Design review of the part built by this model. Coordinates are the model's own, in mm. Face numbers are marked on the shaded views. A direction names the side the tool comes from. Round coordinates to 2 decimals unless told otherwise and drop trailing zeros. Loops run counter-clockwise (first coordinate to the right, second up) from the corner with the lowest first, then second, coordinate; pieces in that order, holes last. Notation, with made-up numbers: (-15, -10.75) - (26, -10.75) arc R34 cw to (26, 20.25) - close; hole circle Ø1 at (80.5, 21). An arc over 180 degrees is marked (long way). Answer as CSV lines item,"result". Start each with the question number.
(1) For the marked faces 4, 5 and 6, list the 3-axis set-ups (+Z, -Z, +X, -X, +Y, -Y) from which the entire face can be reached by the end or side of a thin tool; tool diameter is ignored.
(2) For P1, Ø1.5, axis at x = -2, z = 6, coming from the -Y side; P2, Ø0.6, axis at x = 13, z = 4.5, coming from the -Y side; P3, Ø1.1, axis at x = 1.5, z = 6.5, coming from the +Y side, all flat-tipped, find the tip position at first contact; note any pin that passes through.
(3) Wall thickness on L1, parallel to X at y = 0, z = 1.75; L2, parallel to Y at x = 0, z = 1.25; L3, parallel to Y at x = 0, z = 5.65: over which ranges is each line inside the solid? List them lowest first.
(4) Consider section D-D (x = 5). Give the boundary of the cut face in (y, z), and give its area (3 significant figures).
(5) Consider section B-B (x = 10). Give the boundary of the cut face in (y, z), and give its area (3 significant figures).
(6) Consider section A-A (z = 2). Give the boundary of the cut face in (x, y).
(7) Consider section C-C (x = 0). Give the boundary of the cut face in (y, z) (3 decimals), and give its area (3 significant figures).
(8) Mouldability with a two-part tool opening along Z and no side actions: class the marked faces 1, 2 and 3 as released by +Z, released by -Z, zero draft, split by the parting line, or undercut.
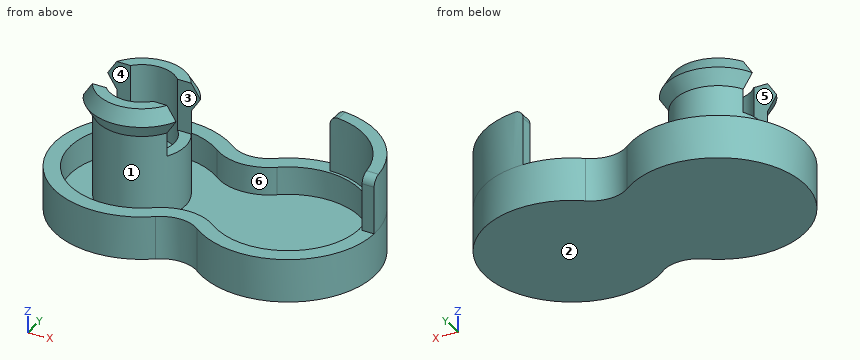
from build123d import *
from build123d.topology import SkipClean

# Parameters (mm, degrees)
BOSS_EXTRUDE1_DEPTH = 2.5
SHELL1_T            = -0.88
BOSS_EXTRUDE2_DEPTH = 3.25
FILLET1_R           = 0.5
FILLET2_R           = 0.5
SKETCH3_R           = 2.5
BOSS_EXTRUDE3_DEPTH = 6.5
SKETCH5_R           = 1.85
CUT_EXTRUDE1_DEPTH  = 4.22
SKETCH8_W           = 6.47168307
SKETCH8_H           = 2.5
CUT_EXTRUDE2_DEPTH  = 3
SKETCH9_W           = 5
SKETCH9_H           = 5
CUT_EXTRUDE3_DEPTH  = 3.25


# Read off the part's stored shape, not the designer's step: Mirror1
with BuildPart() as part:
    # Sketch1 → Boss-Extrude1 (new body)
    with BuildSketch(Plane.XY):
        with BuildLine():
            ThreePointArc((3.035714286, 3.972963475), (-5, 0), (3.035714286, -3.972963475))
            ThreePointArc((3.035714286, -3.972963475), (4.25, -3.562148865), (5.464285714, -3.972963475))
            ThreePointArc((5.464285714, -3.972963475), (13.5, 0), (5.464285714, 3.972963475))
            ThreePointArc((5.464285714, 3.972963475), (4.25, 3.562148865), (3.035714286, 3.972963475))
        make_face()
    extrude(amount=BOSS_EXTRUDE1_DEPTH)

    # Shell1
    shell1_openings = [part.faces().sort_by_distance(p)[0] for p in [
        (4.25, 0, 2.5),
    ]]
    offset(amount=SHELL1_T, openings=shell1_openings, kind=Kind.INTERSECTION)

    # Sketch2 → Boss-Extrude2 (add)
    with BuildSketch(Plane.XY.offset(2.5)):
        with BuildLine():
            Line((13.5, 0), (12.8, 0))
            ThreePointArc((12.8, 0), (11.540559159, -3.040559159), (8.5, -4.3))
            Line((8.5, -4.3), (8.5, -5))
            ThreePointArc((8.5, -5), (12.035533906, -3.535533906), (13.5, 0))
        make_face()
    extrude(amount=BOSS_EXTRUDE2_DEPTH)

    # Fillet1
    fillet1_edges = [part.edges().sort_by_distance(p)[0] for p in [
        (8.5, -4.65, 5.75),
    ]]
    fillet(fillet1_edges, radius=FILLET1_R)

    # Fillet2
    fillet2_edges = [part.edges().sort_by_distance(p)[0] for p in [
        (13.15, 0, 5.75),
    ]]
    fillet(fillet2_edges, radius=FILLET2_R)

    # Sketch3 → Boss-Extrude3 (add)
    with BuildSketch(Plane.XY.offset(0.88)):
        with Locations(Location((0, 0, 0), (0, 0, 180))):
            Circle(SKETCH3_R)
    extrude(amount=BOSS_EXTRUDE3_DEPTH)

    # Sketch5 → Cut-Extrude1 (cut)
    with BuildSketch(Plane.XY.offset(7.38)):
        Circle(SKETCH5_R)
    extrude(amount=-CUT_EXTRUDE1_DEPTH, mode=Mode.SUBTRACT)

    # Sketch6 → Revolve1 (revolve)
    with BuildSketch(Plane(origin=(0, 0, 0), x_dir=(1, 0, 0), z_dir=(0, 1, 0))):
        Polygon((2.5, -5.75), (2.5, -7.38), (2.970540469, -6.565), align=None)
    revolve(axis=Axis((0, 0, 7.38), (0, 0, -1)))

    # Sketch8 → Cut-Extrude2 (cut)
    with BuildSketch(Plane.XY.offset(7.38)):
        Rectangle(SKETCH8_W, SKETCH8_H)
    extrude(amount=-CUT_EXTRUDE2_DEPTH, mode=Mode.SUBTRACT)

    # Mirror1: part across plane


with BuildPart() as part_1:
    with SkipClean():  # the faces are left unmerged after this step: merging them gives an invalid solid
        add(part.part)
        add(part.part.mirror(Plane.ZX))

    # Sketch9 → Cut-Extrude3 (cut)
    with SkipClean():  # the faces are left unmerged after this step: merging them gives an invalid solid
        with BuildSketch(Plane.XY.offset(5.75)):
            with Locations((11, -2.5)):
                Rectangle(SKETCH9_W, SKETCH9_H)
        extrude(amount=-CUT_EXTRUDE3_DEPTH, mode=Mode.SUBTRACT)


solid = part_1.part
Determined:
1,face 4,"+Z, -X"
1,face 5,"+Z, +X, -X"
1,face 6,"+Z"
2,P1,"stops at y = -2.56"
2,P2,"stops at y = 0"
2,P3,"stops at y = 2.81"
3,L1,"x = -5 to -4.12, -2.5 to 2.5, 12.62 to 13.5"
3,L2,"y = -5 to -4.12, -2.5 to 2.5, 4.12 to 5"
3,L3,"y = -2.5 to -1.85, 1.85 to 2.5"
4,outline,"(-3.71, 0) - (3.71, 0) - (3.71, 2.5) - (2.78, 2.5) - (2.78, 0.88) - (-2.78, 0.88) - (-2.78, 2.5) - (-3.71, 2.5) - close"
4,area,"9.53 mm^2"
5,outline,"(-4.77, 0) - (4.77, 0) - (4.77, 5.75) - (4.03, 5.75) - (4.03, 2.5) - (3.84, 2.5) - (3.84, 0.88) - (-3.84, 0.88) - (-3.84, 2.5) - (-4.77, 2.5) - close"
5,area,"13.8 mm^2"
6,outline,"circle Ø5 at (0, 0); (3.04, -3.97) arc R2 cw to (5.46, -3.97) arc R5 ccw (long way) to (5.46, 3.97) arc R2 cw to (3.04, 3.97) arc R5 ccw (long way) to start; hole (2.5, -3.27) arc R2.88 cw to (6, -3.27) arc R4.12 ccw (long way) to (6, 3.27) arc R2.88 cw to (2.5, 3.27) arc R4.12 ccw (long way) to start"
7,outline,"(-5, 0) - (5, 0) - (5, 2.5) - (4.12, 2.5) - (4.12, 0.88) - (2.5, 0.88) - (2.5, 5.75) - (2.971, 6.565) - (2.5, 7.38) - (1.85, 7.38) - (1.85, 3.16) - (-1.85, 3.16) - (-1.85, 7.38) - (-2.5, 7.38) - (-2.971, 6.565) - (-2.5, 5.75) - (-2.5, 0.88) - (-4.12, 0.88) - (-4.12, 2.5) - (-5, 2.5) - close"
7,area,"29.3 mm^2"
8,face 1,"undercut"
8,face 2,"released by -Z"
8,face 3,"zero draft"
